from build123d import *

# Parameters (mm, degrees)
SKETCH1_R                  = 37.5
SKETCH1_R_2                = 35
BOSS_EXTRUDE1_DEPTH        = 345
SKETCH2_R                  = 35.5
SKETCH2_R_2                = 33.5
CUT_EXTRUDE1_DEPTH         = 20
SKETCH3_R                  = 5
CUT_EXTRUDE2_DEPTH         = 10
CUT_EXTRUDE2_DEPTH_BACK    = 30
SKETCH5_R                  = 7
SKETCH5_R_2                = 5
BOSS_EXTRUDE3_DEPTH        = 1
BOSS_EXTRUDE3_2_DEPTH      = 1
SKETCH6_R                  = 7
SKETCH6_R_2                = 5
BOSS_EXTRUDE5_DEPTH        = 1
BOSS_EXTRUDE7_DEPTH        = 50
BOSS_EXTRUDE7_DEPTH_BACK   = 10
BOSS_EXTRUDE7_2_DEPTH      = 50
BOSS_EXTRUDE7_2_DEPTH_BACK = 10
SKETCH13_R                 = 7
SKETCH13_W                 = 40
SKETCH13_H                 = 24.419709383
CUT_EXTRUDE7_DEPTH         = 21
SKETCH14_R                 = 35
CUT_EXTRUDE8_DEPTH         = 346.0000001
SKETCH15_R                 = 7
BOSS_EXTRUDE8_DEPTH        = 8
SKETCH16_W                 = 40
SKETCH16_H                 = 24.419709383
CUT_EXTRUDE11_DEPTH        = 97
FILLET1_R                  = 2
FILLET2_R                  = 2
BOSS_EXTRUDE12_DEPTH       = 40


with BuildPart() as part:
    # Sketch1 → Boss-Extrude1 (new body)
    with BuildSketch(Plane(origin=(0, 0, 0), x_dir=(1, 0, 0), z_dir=(0, 1, 0))):
        Circle(SKETCH1_R)
        Circle(SKETCH1_R_2, mode=Mode.SUBTRACT)
    extrude(amount=BOSS_EXTRUDE1_DEPTH)

    # Sketch2 → Cut-Extrude1 (cut)
    with BuildSketch(Plane.XZ):
        Circle(SKETCH2_R)
        Circle(SKETCH2_R_2, mode=Mode.SUBTRACT)
    extrude(amount=-CUT_EXTRUDE1_DEPTH, mode=Mode.SUBTRACT)

    # Sketch3 → Cut-Extrude2 (cut, two sides)
    with BuildSketch(Plane.XY.offset(36.5)) as cut_extrude2_sk:
        with Locations((0, 120)):
            Circle(SKETCH3_R)
        with Locations((0, 90)):
            Circle(SKETCH3_R)
        with Locations((0, 150)):
            Circle(SKETCH3_R)
    extrude(amount=CUT_EXTRUDE2_DEPTH, mode=Mode.SUBTRACT)
    extrude(cut_extrude2_sk.sketch, amount=-CUT_EXTRUDE2_DEPTH_BACK, mode=Mode.SUBTRACT)



with BuildPart() as body_2:
    # Sketch5 → Boss-Extrude3 (new body)
    with BuildSketch(Plane.XY.offset(36.5)):
        with Locations((0, 120)):
            Circle(SKETCH5_R)
        with Locations((0, 120)):
            Circle(SKETCH5_R_2, mode=Mode.SUBTRACT)
    extrude(amount=-BOSS_EXTRUDE3_DEPTH)


with BuildPart() as body_3:
    # Sketch5 → Boss-Extrude3 2 (new body)
    with BuildSketch(Plane.XY.offset(36.5)):
        with Locations((0, 90)):
            Circle(SKETCH5_R)
        with Locations((0, 90)):
            Circle(SKETCH5_R_2, mode=Mode.SUBTRACT)
    extrude(amount=-BOSS_EXTRUDE3_2_DEPTH)


with BuildPart() as part_1:
    add(part.part)

    add(body_2.part)  # Boss-Extrude5 merges body 2

    add(body_3.part)  # Boss-Extrude5 merges body 3
    # Sketch6 → Boss-Extrude5 (add)
    with BuildSketch(Plane.XY.offset(36.5)):
        with Locations((0, 120)):
            Circle(SKETCH6_R)
        with Locations((0, 120)):
            Circle(SKETCH6_R_2, mode=Mode.SUBTRACT)
        with Locations((0, 150)):
            Circle(SKETCH6_R)
        with Locations((0, 150)):
            Circle(SKETCH6_R_2, mode=Mode.SUBTRACT)
        with Locations((0, 90)):
            Circle(SKETCH6_R)
        with Locations((0, 90)):
            Circle(SKETCH6_R_2, mode=Mode.SUBTRACT)
    extrude(amount=BOSS_EXTRUDE5_DEPTH)



with BuildPart() as body_2_2:
    # Sketch12 → Boss-Extrude7 (new body, two sides)
    with BuildSketch(Plane(origin=(0, 0, -37.5), x_dir=(-1, 0, 0), z_dir=(0, 0, -1))) as boss_extrude7_sk:
        Polygon((20, 165), (0, 165), (-20, 165), (-20, 170), (20, 170), align=None)
    extrude(amount=BOSS_EXTRUDE7_DEPTH)
    extrude(boss_extrude7_sk.sketch, amount=-BOSS_EXTRUDE7_DEPTH_BACK)

    # Sketch13 → Cut-Extrude7 (cut)
    with BuildSketch(Plane(origin=(0, 170, 0), x_dir=(1, 0, 0), z_dir=(0, 1, 0))):
        with Locations((0, 51.13401188)):
            Circle(SKETCH13_R)
        with Locations((0, 75.290145309)):
            Rectangle(SKETCH13_W, SKETCH13_H)
    extrude(amount=-CUT_EXTRUDE7_DEPTH, mode=Mode.SUBTRACT)


with BuildPart() as body_3_2:
    # Sketch12 → Boss-Extrude7 2 (new body, two sides)
    with BuildSketch(Plane(origin=(0, 0, -37.5), x_dir=(-1, 0, 0), z_dir=(0, 0, -1))) as boss_extrude7_2_sk:
        Polygon((20, 135), (20, 130), (0, 130), (-20, 130), (-20, 135), align=None)
    extrude(amount=BOSS_EXTRUDE7_2_DEPTH)
    extrude(boss_extrude7_2_sk.sketch, amount=-BOSS_EXTRUDE7_2_DEPTH_BACK)


with BuildPart() as cut_extrude8_tool:
    # Sketch14 → Cut-Extrude8 (new body, through all)
    with BuildSketch(Plane(origin=(0, 345, 0), x_dir=(1, 0, 0), z_dir=(0, 1, 0))):
        Circle(SKETCH14_R)
    extrude(amount=-CUT_EXTRUDE8_DEPTH)


with BuildPart() as body_2_2_1:
    add(body_2_2.part)

    # Cut-Extrude8: cut by cut_extrude8_tool
    add(cut_extrude8_tool.part, mode=Mode.SUBTRACT)

    # Sketch15 → Boss-Extrude8 (add)
    with BuildSketch(Plane(origin=(0, 170, 0), x_dir=(1, 0, 0), z_dir=(0, 1, 0))):
        Polygon((11.547005384, 51.13401188), (5.773502692, 61.13401188), (-5.773502692, 61.13401188), (-11.547005384, 51.13401188), (-5.773502692, 41.13401188), (5.773502692, 41.13401188), align=None)
        with Locations((0, 51.13401188)):
            Circle(SKETCH15_R, mode=Mode.SUBTRACT)
    extrude(amount=BOSS_EXTRUDE8_DEPTH)

    # Fillet1
    fillet1_edges = [body_2_2_1.edges().sort_by_distance(p)[0] for p in [
        (20, 167.5, -63.080290617),
        (-20, 167.5, -63.080290617),
    ]]
    fillet(fillet1_edges, radius=FILLET1_R)


with BuildPart() as body_3_2_1:
    add(body_3_2.part)

    # Cut-Extrude8: cut by cut_extrude8_tool
    add(cut_extrude8_tool.part, mode=Mode.SUBTRACT)

    # Sketch16 → Cut-Extrude11 (cut)
    with BuildSketch(Plane(origin=(0, 170, 0), x_dir=(1, 0, 0), z_dir=(0, 1, 0))):
        with Locations((0, 75.290145309)):
            Rectangle(SKETCH16_W, SKETCH16_H)
    extrude(amount=-CUT_EXTRUDE11_DEPTH, mode=Mode.SUBTRACT)

    # Fillet2
    fillet2_edges = [body_3_2_1.edges().sort_by_distance(p)[0] for p in [
        (20, 132.5, -63.080290617),
        (-20, 132.5, -63.080290617),
    ]]
    fillet(fillet2_edges, radius=FILLET2_R)


with BuildPart() as part_2:
    add(part_1.part)

    add(body_2_2_1.part)  # Boss-Extrude12 merges body 2 2

    add(body_3_2_1.part)  # Boss-Extrude12 merges body 3 2
    # Sketch18 → Boss-Extrude12 (add)
    with BuildSketch(Plane(origin=(20, 0, 0), x_dir=(0, 0, -1), z_dir=(1, 0, 0))):
        Polygon((39.490080652, 165), (37.410474121, 165), (36.415879692, 165), (36.415879692, 135), (39.490080652, 135), align=None)
    extrude(amount=-BOSS_EXTRUDE12_DEPTH)


solid = part_2.part
Design review of the part built by this model. Coordinates are the model's own, in mm. A direction names the side the tool comes from. Give positions to 0.01 mm unless a question says otherwise; leave off trailing zeros. Order: outer loops, then holes, each group sorted by start corner. A loop starts at its lowest first (then second) coordinate and runs counter-clockwise, first axis right, second up. Notation, with made-up numbers: (-14.5, 50) - (25.5, 50) arc R24 cw to (25.5, 77) - close; hole circle Ø5 at (35.5, -5.5). An arc over 180 degrees is marked (long way). Write item = value, one per line. Start each with the question number.
Q1. Mouldability with a two-part tool opening along Z and no side actions: class faces 1 (the face through (-7.696, 9.86, -34.656)), 2 (the face through (2, 178, -58)), 3 (the face through (-2, 125, 37.5)), 4 (the face through (-14, 150, -36.416)) as released by +Z, released by -Z, zero draft, split by the parting line, or undercut.
Q2. To check wall thickness, follow L1, parallel to Y at x = 0, z = 36; L2, parallel to Z at x = 0, y = 168; L3, parallel to Z at x = 0, y = 189. State the ranges of each line that lie inside material, in increasing order. Write a range as from..to.
Q3. We need section B-B on x = -26. State the section outline as (y, z) points.
Q4. We need section D-D on y = 47. State the section outline as (x, z) points, plus the area to 3 significant figures.
Q5. We need section C-C on y = 150. State the section outline as (x, z) points.
Q6. We need section A-A on z = 0. State the section outline as (x, y) points.
Q7. Clearance check with flat-ended pins moving along their axes: pin 1 Ø1.5 at (y, z) = (196.5, 11.5) entering from +X; pin 2 Ø6 at (x, y) = (-9, 57) entering from +Z; pin 3 Ø12 at (x, z) = (-6.5, -52) entering from +Y; pin 4 Ø14.5 at (y, z) = (157, -53) entering from +X. State where each tip first meets the part, or that it passes through.
Q8. Tool access review of faces 5 (the face through (0, 174, -41.134)), 6 (the face through (0, 174, -61.134)), 7 (the face through (-20, 149, -39)), 8 (the face through (8.62, 173.944, -46.064)), 9 (the face through (0, 150, -39.49)): name each direction out of +Z, -Z, +X, -X, +Y, -Y from which nothing blocks a thin tool from reaching the whole face with its end or side.
Working result:
q1.face_1 = undercut
q1.face_2 = zero draft
q1.face_3 = released by +Z
q1.face_4 = undercut
q2.L1 = 0..85, 95..115, 125..145, 155..345
q2.L2 = -63.08..-58.13, -44.13..-35, 35..37.5
q2.L3 = -37.5..-35, 35..37.5
q3.outline = (0, -27.02) - (345, -27.02) - (345, -23.43) - (20, -23.43) - (20, -24.17) - (0, -24.17) - close; (0, 24.17) - (20, 24.17) - (20, 23.43) - (345, 23.43) - (345, 27.02) - (0, 27.02) - close
q4.outline = circle Ø75 at (0, 0); hole circle Ø70 at (0, 0)
q4.area = 569 mm²
q5.outline = (-20, -39.49) - (20, -39.49) - (20, -36.42) - (8.95, -36.42) arc R37.5 ccw to (7, 36.84) - (7, 37.5) - (5, 37.5) - (5, 34.64) arc R35 cw (long way) to (-5, 34.64) - (-5, 37.5) - (-7, 37.5) - (-7, 36.84) arc R37.5 ccw to (-8.95, -36.42) - (-20, -36.42) - close
q6.outline = (-37.5, 0) - (-35.5, 0) - (-35.5, 20) - (-35, 20) - (-35, 345) - (-37.5, 345) - close; (35, 20) - (35.5, 20) - (35.5, 0) - (37.5, 0) - (37.5, 345) - (35, 345) - close
q7.pin_1 = 35.93
q7.pin_2 = 37.02
q7.pin_3 = 178
q7.pin_4 = through
q8.face_5 = +X, -X, +Y
q8.face_6 = -Z, +X, -X, +Y
q8.face_7 = -Z, -X, +Y, -Y
q8.face_8 = +X, +Y
q8.face_9 = -Z, +X, -X
